from build123d import *

# Parameters (mm, degrees)
SALIENTE_EXTRUIR1_DEPTH = 80
CROQUIS2_W              = 3
CROQUIS2_H              = 15
SALIENTE_EXTRUIR2_DEPTH = 3
CROQUIS3_W              = 3
CROQUIS3_H              = 15
SALIENTE_EXTRUIR3_DEPTH = 3
CORTAR_EXTRUIR1_DEPTH   = 10
CROQUIS5_W              = 10
CROQUIS5_H              = 3
SALIENTE_EXTRUIR4_DEPTH = 3


with BuildPart() as part:
    # Croquis1 → Saliente-Extruir1 (new body)
    with BuildSketch(Plane.XY):
        Polygon((3, 0), (3, -63.5), (0, -66.017298894), (0, 0), (0, 10), (3, 10), align=None)
    extrude(amount=SALIENTE_EXTRUIR1_DEPTH)

    # Croquis2 → Saliente-Extruir2 (add)
    with BuildSketch(Plane.XY.offset(80)):
        with Locations((1.5, -17.5)):
            Rectangle(CROQUIS2_W, CROQUIS2_H)
        with Locations((1.5, -42.5)):
            Rectangle(CROQUIS2_W, CROQUIS2_H)
    extrude(amount=SALIENTE_EXTRUIR2_DEPTH)

    # Croquis3 → Saliente-Extruir3 (add)
    with BuildSketch(Plane(origin=(0, 0, 0), x_dir=(-1, 0, 0), z_dir=(0, 0, -1))):
        with Locations((-1.5, -17.5)):
            Rectangle(CROQUIS3_W, CROQUIS3_H)
        with Locations((-1.5, -42.5)):
            Rectangle(CROQUIS3_W, CROQUIS3_H)
    extrude(amount=SALIENTE_EXTRUIR3_DEPTH)

    # Croquis4 → Cortar-Extruir1 (cut)
    with BuildSketch(Plane.ZY):
        Polygon((0, 1.5), (8, 1.5), (8, 3.5), (11, 3.5), (11, 1.5), (15, 1.5), (15, -1.5), (11, -1.5), (11, -3.5), (8, -3.5), (8, -1.5), (0, -1.5), align=None)
        Polygon((69, -1.5), (65, -1.5), (65, 1.5), (69, 1.5), (69, 3.5), (72, 3.5), (72, 1.5), (80, 1.5), (80, -1.5), (72, -1.5), (72, -3.5), (69, -3.5), align=None)
    extrude(amount=-CORTAR_EXTRUIR1_DEPTH, mode=Mode.SUBTRACT)

    # Croquis5 → Saliente-Extruir4 (add)
    with BuildSketch(Plane.ZY):
        with Locations((20, 11.5)):
            Rectangle(CROQUIS5_W, CROQUIS5_H)
        with Locations((60, 11.5)):
            Rectangle(CROQUIS5_W, CROQUIS5_H)
    extrude(amount=-SALIENTE_EXTRUIR4_DEPTH)


solid = part.part
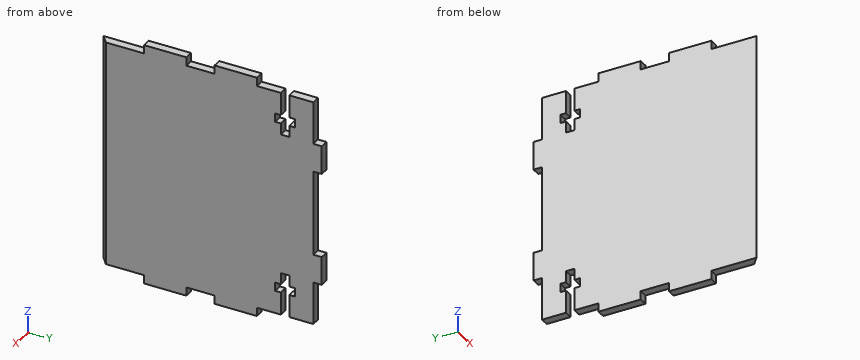
CAD build for the part. Positions are in the model's coordinates, mm. Round coordinates to 2 decimals unless told otherwise and drop trailing zeros. Write each loop counter-clockwise with the first axis right and the second up, starting at its lowest first coordinate (ties: lowest second). Pieces come first, ordered by that corner, then holes. Notation, with made-up numbers: (-40, 52.5) -> (-20, 52.5) arc R13 ccw to (-20, 56.5) -> close; hole circle Ø5 at (39.5, 25.25). An arc over 180 degrees is marked (long way). Answer as a JSON object with one key per item and string values.
(1) Band-saw the part on B-B, the plane z = 36. List the corners of the cut face in (x, y), then the cut area to 3 significant figures.
Reported:
{"outline": "(0, -66.02) -> (3, -63.5) -> (3, 10) -> (0, 10) -> close", "area": "224 mm^2"}
(2) Pin check, flat tips, straight feed: P1, Ø1.5, axis at x = 1, z = 9, coming from the +Y side; P2, Ø8, axis at y = -29, z = 42.5, coming from the -X side; P3, Ø1.5, axis at x = 1, y = -6.5, coming from the -Z side; P4, Ø1.6, axis at x = 1.5, y = -3, coming from the +Z side. Stop position of each tip, or through.
Reported:
{"P1": "stops at y = 10", "P2": "stops at x = 0", "P3": "stops at z = 0", "P4": "stops at z = 80"}
(3) Probe probe 1 along Z at (x, y) = (1.8, 3); probe 2 along Z at (x, y) = (2.1, -26); probe 3 along Y at (x, z) = (1.1, 70.5). List the from-to ranges inside material, lowest first. Write a range as [from, to].
Reported:
{"probe 1": "z = [0, 8], [11, 69], [72, 80]", "probe 2": "z = [0, 80]", "probe 3": "y = [-65.09, -3.5], [3.5, 10]"}
(4) Band-saw the part on A-A, the plane z = 3. List the corners of the cut face in (x, y).
Reported:
{"outline": "(0, -66.02) -> (3, -63.5) -> (3, -1.5) -> (0, -1.5) -> close; (0, 1.5) -> (3, 1.5) -> (3, 10) -> (0, 10) -> close"}
(5) Band-saw the part on C-C, the plane y = -54. List the corners of the cut face in (x, z).
Reported:
{"outline": "(0, 0) -> (3, 0) -> (3, 80) -> (0, 80) -> close"}
